from build123d import *

# Parameters (mm, degrees)
F0_W     = 24.553348
F0_H     = 25.4
F1_DEPTH = 25.4
F2_R     = 2.54
F3_DEPTH = 25.4
F4_R     = 2.54
F5_W     = 6.35
F5_H     = 16.256
F6_DEPTH = 25.4
F7_W     = 6.35
F7_H     = 8.128
F9_DEPTH = 25.4


with BuildPart() as f1:
    # F0 (on Top) → F1 (new body)
    with BuildSketch(Plane.XY):
        Rectangle(F0_W, F0_H)
    extrude(amount=F1_DEPTH)

    # F2 (on face) → F3 (cut)
    with BuildSketch(Plane.XY.offset(25.4)):
        Circle(F2_R)
    extrude(amount=-F3_DEPTH, mode=Mode.SUBTRACT)

    # F4
    f4_edges = [f1.edges().sort_by_distance(p)[0] for p in [
        (-12.276674, -12.7, 12.7),
        (-12.276674, 12.7, 12.7),
        (12.276674, -12.7, 12.7),
        (12.276674, 12.7, 12.7),
    ]]
    fillet(f4_edges, radius=F4_R)

    # F5 (on face) → F6 (cut)
    with BuildSketch(Plane.XY.offset(25.4)):
        with Locations((0, 12.7)):
            Rectangle(F5_W, F5_H)
    extrude(amount=-F6_DEPTH, mode=Mode.SUBTRACT)

    # F7 (on face) → F9 (cut)
    with BuildSketch(Plane.XY.offset(25.4)):
        with Locations((0, 8.636)):
            Rectangle(F7_W, F7_H)
        Polygon((-3.175, -4.572), (-3.175001, -12.7), (3.174999, -12.7), (3.175, -4.572), align=None)
    extrude(amount=-F9_DEPTH, mode=Mode.SUBTRACT)


solid = f1.part
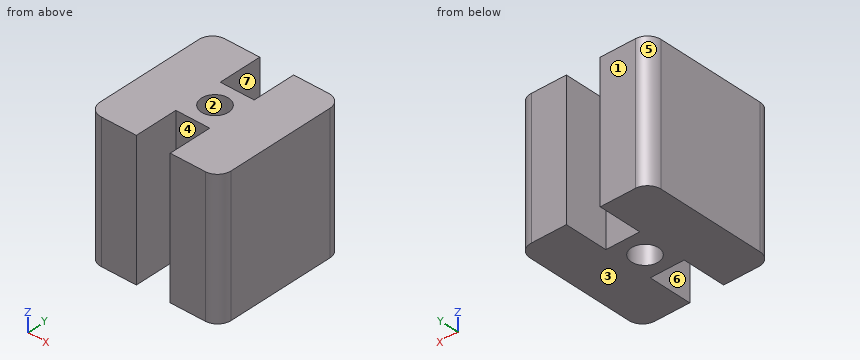
Read the model definition and answer for the solid it produces. Units are mm, in the model's axes. Face numbers are marked on the shaded views. A direction names the side the tool comes from. Give positions to 0.01 mm unless a question says otherwise; leave off trailing zeros. Write each loop counter-clockwise with the first axis right and the second up, starting at its lowest first coordinate (ties: lowest second). Pieces come first, ordered by that corner, then holes. Notation, with made-up numbers: (-28.5, 21.5) -> (2.5, 21.5) arc R21 cw to (2.5, 34.5) -> close; hole circle Ø4 at (57, -14.5). An arc over 180 degrees is marked (long way). Answer as a JSON object with one key per item and string values. Group by question number.
1) This flat-tipped pin is pushed along its axis until it touches: P1, Ø3, axis at x = 1, z = 15, coming from the -Y side. Where does it stop, or does it pass through?
2) Consider L1, parallel to Y at x = 0, z = 15.25; L2, parallel to X at y = -1.75, z = 23.5; L3, parallel to Y at x = 10.75, z = 11. Determine where each line is inside the solid, lowest interval first. Write a range as from..to.
3) Find section B-B (x = 0). Write down the section's boundary in (y, z), and give its area (3 significant figures).
4) Find section A-A (y = 0). Write down the section's boundary in (x, z).
5) A tool of negligible diameter and unlimited length cuts with its end or side. For the marked faces 5, 6 and 7, from which of +Z, -Z, +X, -X, +Y, -Y can it reach the whole face along a straight path? Write none if from no direction.
6) The mould has two halves that part along Y. Classify the marked faces 1, 2, 3 and 4: +Y half, -Y half, draft (parallel to the pull), parting line (faces both ways), or undercut.
7) Find section C-C (z = 3.5). Write down the section's boundary in (x, y) (3 decimals), and give its area (3 significant figures).
Values follow:
{
 "1": {"P1": "stops at y = -4.57"},
 "2": {"L1": "y = -4.57..-2.54, 2.54..4.57", "L2": "x = -12.28..-1.84, 1.84..12.28", "L3": "y = -12.49..12.49"},
 "3": {"outline": "(-4.57, 0) -> (-2.54, 0) -> (-2.54, 25.4) -> (-4.57, 25.4) -> close; (2.54, 0) -> (4.57, 0) -> (4.57, 25.4) -> (2.54, 25.4) -> close", "area": "103 mm2"},
 "4": {"outline": "(-12.28, 0) -> (-2.54, 0) -> (-2.54, 25.4) -> (-12.28, 25.4) -> close; (2.54, 0) -> (12.28, 0) -> (12.28, 25.4) -> (2.54, 25.4) -> close"},
 "5": {"face 5": "+Z, -Z, -X, +Y", "face 6": "+Z, -Z, -Y", "face 7": "+Z, -Z, +Y"},
 "6": {"face 1": "+Y half", "face 2": "undercut", "face 3": "draft", "face 4": "-Y half"},
 "7": {"outline": "(-12.277, -10.16) arc R2.54 ccw to (-9.737, -12.7) -> (-3.175, -12.7) -> (-3.175, -4.572) -> (3.175, -4.572) -> (3.175, -12.7) -> (9.737, -12.7) arc R2.54 ccw to (12.277, -10.16) -> (12.277, 10.16) arc R2.54 ccw to (9.737, 12.7) -> (3.175, 12.7) -> (3.175, 4.572) -> (-3.175, 4.572) -> (-3.175, 12.7) -> (-9.737, 12.7) arc R2.54 ccw to (-12.277, 10.16) -> close; hole circle Ø5.08 at (0, 0)", "area": "495 mm2"}
}
